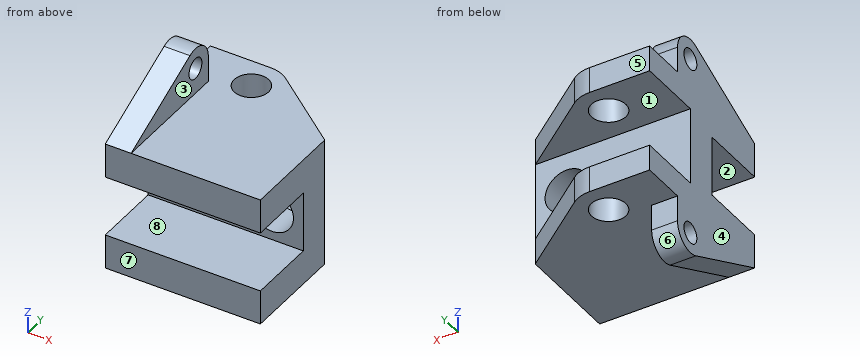
```python
from build123d import *

# Parameters (mm, degrees)
BOSS_EXTRUDE1_DEPTH = 90
SKETCH2_R           = 10
BOSS_EXTRUDE2_DEPTH = 15
BOSS_EXTRUDE3_START = -15
SKETCH3_R           = 10
BOSS_EXTRUDE3_DEPTH = 15
SKETCH5_R           = 6
BOSS_EXTRUDE4_DEPTH = 15
SKETCH6_R           = 6
BOSS_EXTRUDE5_DEPTH = 15
SKETCH7_R           = 12.5
CUT_EXTRUDE1_DEPTH  = 133.315560912


with BuildPart() as part:
    # Sketch1 → Boss-Extrude1 (new body)
    with BuildSketch(Plane(origin=(0, 0, 0), x_dir=(0, 0, -1), z_dir=(1, 0, 0))):
        Polygon((-25.793650794, 0), (-25.793650794, 60), (49.206349206, 60), (49.206349206, 0), (29.206349206, 0), (29.206349206, 40), (-5.793650794, 40), (-5.793650794, 0), align=None)
    extrude(amount=-BOSS_EXTRUDE1_DEPTH)

    # Sketch2 → Boss-Extrude2 (add)
    with BuildSketch(Plane.XY.offset(25.793650794)):
        with BuildLine():
            Line((0, 60), (-43.943887784, 94.204308595))
            ThreePointArc((-43.943887784, 94.204308595), (-49.155239727, 97.024652048), (-55, 98))
            Line((-55, 98), (-90, 98))
            Line((-90, 98), (-90, 60))
            Line((-90, 60), (0, 60))
        make_face()
        with Locations((-55, 80)):
            Circle(SKETCH2_R, mode=Mode.SUBTRACT)
    extrude(amount=-BOSS_EXTRUDE2_DEPTH)

    # Sketch3 → Boss-Extrude3 (add)
    with BuildSketch(Plane(origin=(0, 0, -49.206349206), x_dir=(-1, 0, 0), z_dir=(0, 0, -1)).offset(BOSS_EXTRUDE3_START)):
        with BuildLine():
            Line((0, 60), (90, 60))
            Line((90, 60), (90, 98))
            Line((90, 98), (55, 98))
            ThreePointArc((55, 98), (49.155239727, 97.024652048), (43.943887784, 94.204308595))
            Line((43.943887784, 94.204308595), (0, 60))
        make_face()
        with Locations(Location((55, 80, 0), (0, 0, 180))):
            Circle(SKETCH3_R, mode=Mode.SUBTRACT)
    extrude(amount=BOSS_EXTRUDE3_DEPTH)

    # Sketch5 → Boss-Extrude4 (add)
    with BuildSketch(Plane.ZY.offset(90)):
        with BuildLine():
            Line((25.793650794, 0), (25.793650794, 72))
            Line((25.793650794, 72), (40.793650794, 72))
            ThreePointArc((40.793650794, 72), (50.926944716, 66.427779888), (51.649414605, 54.886059047))
            Line((51.649414605, 54.886059047), (25.793650794, 0))
        make_face()
        with Locations((40.793650794, 60)):
            Circle(SKETCH5_R, mode=Mode.SUBTRACT)
    extrude(amount=-BOSS_EXTRUDE4_DEPTH)

    # Sketch6 → Boss-Extrude5 (add)
    with BuildSketch(Plane.ZY.offset(90)):
        with BuildLine():
            Line((-49.206349206, 0), (-75.062113018, 54.886059047))
            ThreePointArc((-75.062113018, 54.886059047), (-74.339643129, 66.427779888), (-64.206349206, 72))
            Line((-64.206349206, 72), (-49.206349206, 72))
            Line((-49.206349206, 72), (-49.206349206, 0))
        make_face()
        with Locations((-64.206349206, 60)):
            Circle(SKETCH6_R, mode=Mode.SUBTRACT)
    extrude(amount=-BOSS_EXTRUDE5_DEPTH)

    # Sketch7 → Cut-Extrude1 (cut, through all)
    with BuildSketch(Plane(origin=(0, 60, 0), x_dir=(1, 0, 0), z_dir=(0, 1, 0))):
        with Locations(Location((-18.195009626, 11.706349206, 0), (0, 0, 270))):
            Circle(SKETCH7_R)
    extrude(amount=-CUT_EXTRUDE1_DEPTH, mode=Mode.SUBTRACT)


solid = part.part
```
CAD build for the part. Positions are in the model's coordinates, mm. Face numbers are marked on the shaded views. A direction names the side the tool comes from. Coordinates: 2 decimals unless noted, no trailing zeros. Write each loop counter-clockwise with the first axis right and the second up, starting at its lowest first coordinate (ties: lowest second). Pieces come first, ordered by that corner, then holes.
(1) Flat gauge pins, fed straight in: pin 1 (12 mm diameter, centred on x = -13.5, y = 58, fed in from +Z); pin 2 (19 mm diameter, centred on x = -43, y = 78.5, fed in from -Z); pin 3 (8 mm diameter, centred on y = 26.5, z = 42, fed in from +X). Where does each tip first touch, or does it go through?
(2) Cut at D-D, the plane z = 23.5. List the corners of the cut face in (x, y), and give its area (3 significant figures).
(3) 3-axis set-ups, long thin cutter, end or side, ignore diameter. For the marked faces 1, 2, 3, 4 and 5: which of +Z, -Z, +X, -X, +Y, -Y reach the whole face in a straight line?
(4) Drill centre lines: probe 1 along Y at (x, z) = (-55, -42); probe 2 along Z at (x, y) = (-66, 13); probe 3 along Z at (x, y) = (-57, 67). Where is each one in solid material? Low to high.
(5) Cut at A-A, the plane z = -62. List the corners of the cut face in (x, y).
(6) Cut at C-C, the plane y = 32. List the corners of the cut face in (x, z).
(7) Two-plate mould, pull along Z, no slides. Class the marked faces 6, 7 and 8: +Z half, -Z half, draft (parallel to the pull), parting line (faces both ways), or undercut.
(8) Cut at B-B, the plane x = -82. List the corners of the cut face in (y, z), and give its area (3 significant figures).
Geometry says:
1. pin 1: stops at z = 25.79
1. pin 2: stops at z = -49.21
1. pin 3: stops at x = -75
2. outline: (-90, 0) - (0, 0) - (0, 60) - (-43.94, 94.2) arc R18 ccw to (-55, 98) - (-90, 98) - close; hole circle Ø20 at (-55, 80)
2. area: 7,570 mm2
3. face 1: +X, -X, +Y
3. face 2: +X, -X, -Y
3. face 3: +Z, +X, +Y, -Y
3. face 4: +Z, -Z, -X, +Y, -Y
3. face 5: +Z, -Z, +X, -X, +Y
4. probe 1: y = 0 to 70, 90 to 98
4. probe 2: z = -49.21 to -29.21, 5.79 to 25.79
4. probe 3: z = -49.21 to -34.21, 10.79 to 25.79
5. outline: (-90, 27.16) - (-75, 27.16) - (-75, 54.42) - (-90, 54.42) - close; (-90, 65.58) - (-75, 65.58) - (-75, 72) - (-90, 72) - close
6. outline: (-90, -64.28) - (-75, -64.28) - (-75, -49.21) - (0, -49.21) - (0, -29.21) - (-90, -29.21) - close; (-90, 5.79) - (0, 5.79) - (0, 25.79) - (-75, 25.79) - (-75, 40.87) - (-90, 40.87) - close
7. face 6: -Z half
7. face 7: draft
7. face 8: undercut
8. outline: (0, -49.21) - (54.89, -75.06) arc R12 ccw to (72, -64.21) - (72, -49.21) - (98, -49.21) - (98, -34.21) - (60, -34.21) - (60, 10.79) - (98, 10.79) - (98, 25.79) - (72, 25.79) - (72, 40.79) arc R12 ccw to (54.89, 51.65) - (0, 25.79) - (0, 5.79) - (40, 5.79) - (40, -29.21) - (0, -29.21) - close; hole circle Ø12 at (60, -64.21); hole circle Ø12 at (60, 40.79)
8. area: 6,290 mm2
